from build123d import *

# Parameters (mm, degrees)
ESBO_O1_R                  = 25
EXTRUS_O1_DEPTH            = 8
EXTRUS_O2_DEPTH            = 8
CIRPATTERN1_COUNT          = 16
CORTE_EXTRUS_O2_DEPTH      = 10
CORTE_EXTRUS_O2_DEPTH_BACK = 37.138621999
ESBO_O5_R                  = 1.25
ESBO_O5_R_2                = 6
ESBO_O8_R                  = 23
ESBO_O8_R_2                = 19.75
CORTE_EXTRUS_O4_DEPTH      = 2
ESBO_O9_R                  = 9.5
CORTE_EXTRUS_O5_DEPTH      = 6
ESBO_O10_R                 = 1.5
CORTE_EXTRUS_O6_DEPTH      = 37.138621999


with BuildPart() as part:
    # Esboço1 → Extrusão1 (new body)
    with BuildSketch(Plane.XY):
        Circle(ESBO_O1_R)
    extrude(amount=-EXTRUS_O1_DEPTH)


with BuildPart() as body_2:
    # Esboço2 → Extrusão2 (new, through all)
    with BuildSketch(Plane(origin=(0, 0, -8), x_dir=(-1, 0, 0), z_dir=(0, 0, -1))):
        Polygon((0, 14.5), (2, 14.5), (2, 29.5), (-2, 29.5), (-2, 14.5), align=None)
    extrude(amount=-EXTRUS_O2_DEPTH)


with BuildPart() as cirpattern1_1:
    # CirPattern1: pattern copy
    add(body_2.part.rotate(Axis((0, 0, 0), (0, 0, 1)), 1 * 360 / CIRPATTERN1_COUNT))


with BuildPart() as cirpattern1_2:
    # CirPattern1: pattern copy
    add(body_2.part.rotate(Axis((0, 0, 0), (0, 0, 1)), 2 * 360 / CIRPATTERN1_COUNT))


with BuildPart() as cirpattern1_3:
    # CirPattern1: pattern copy
    add(body_2.part.rotate(Axis((0, 0, 0), (0, 0, 1)), 3 * 360 / CIRPATTERN1_COUNT))


with BuildPart() as cirpattern1_4:
    # CirPattern1: pattern copy
    add(body_2.part.rotate(Axis((0, 0, 0), (0, 0, 1)), 4 * 360 / CIRPATTERN1_COUNT))


with BuildPart() as cirpattern1_5:
    # CirPattern1: pattern copy
    add(body_2.part.rotate(Axis((0, 0, 0), (0, 0, 1)), 5 * 360 / CIRPATTERN1_COUNT))


with BuildPart() as cirpattern1_6:
    # CirPattern1: pattern copy
    add(body_2.part.rotate(Axis((0, 0, 0), (0, 0, 1)), 6 * 360 / CIRPATTERN1_COUNT))


with BuildPart() as cirpattern1_7:
    # CirPattern1: pattern copy
    add(body_2.part.rotate(Axis((0, 0, 0), (0, 0, 1)), 7 * 360 / CIRPATTERN1_COUNT))


with BuildPart() as cirpattern1_8:
    # CirPattern1: pattern copy
    add(body_2.part.rotate(Axis((0, 0, 0), (0, 0, 1)), 8 * 360 / CIRPATTERN1_COUNT))


with BuildPart() as cirpattern1_9:
    # CirPattern1: pattern copy
    add(body_2.part.rotate(Axis((0, 0, 0), (0, 0, 1)), 9 * 360 / CIRPATTERN1_COUNT))


with BuildPart() as cirpattern1_10:
    # CirPattern1: pattern copy
    add(body_2.part.rotate(Axis((0, 0, 0), (0, 0, 1)), 10 * 360 / CIRPATTERN1_COUNT))


with BuildPart() as cirpattern1_11:
    # CirPattern1: pattern copy
    add(body_2.part.rotate(Axis((0, 0, 0), (0, 0, 1)), 11 * 360 / CIRPATTERN1_COUNT))


with BuildPart() as cirpattern1_12:
    # CirPattern1: pattern copy
    add(body_2.part.rotate(Axis((0, 0, 0), (0, 0, 1)), 12 * 360 / CIRPATTERN1_COUNT))


with BuildPart() as cirpattern1_13:
    # CirPattern1: pattern copy
    add(body_2.part.rotate(Axis((0, 0, 0), (0, 0, 1)), 13 * 360 / CIRPATTERN1_COUNT))


with BuildPart() as cirpattern1_14:
    # CirPattern1: pattern copy
    add(body_2.part.rotate(Axis((0, 0, 0), (0, 0, 1)), 14 * 360 / CIRPATTERN1_COUNT))


with BuildPart() as cirpattern1_15:
    # CirPattern1: pattern copy
    add(body_2.part.rotate(Axis((0, 0, 0), (0, 0, 1)), 15 * 360 / CIRPATTERN1_COUNT))


with BuildPart() as part_1:
    add(part.part)

    # Combinar1: cut CirPattern1_15, body 2, CirPattern1_1, CirPattern1_2, CirPattern1_3, CirPattern1_4, CirPattern1_5, CirPattern1_6, CirPattern1_7, CirPattern1_8, CirPattern1_9, CirPattern1_10, CirPattern1_11, CirPattern1_12, CirPattern1_13, CirPattern1_14
    add(cirpattern1_15.part, mode=Mode.SUBTRACT)
    add(body_2.part, mode=Mode.SUBTRACT)
    add(cirpattern1_1.part, mode=Mode.SUBTRACT)
    add(cirpattern1_2.part, mode=Mode.SUBTRACT)
    add(cirpattern1_3.part, mode=Mode.SUBTRACT)
    add(cirpattern1_4.part, mode=Mode.SUBTRACT)
    add(cirpattern1_5.part, mode=Mode.SUBTRACT)
    add(cirpattern1_6.part, mode=Mode.SUBTRACT)
    add(cirpattern1_7.part, mode=Mode.SUBTRACT)
    add(cirpattern1_8.part, mode=Mode.SUBTRACT)
    add(cirpattern1_9.part, mode=Mode.SUBTRACT)
    add(cirpattern1_10.part, mode=Mode.SUBTRACT)
    add(cirpattern1_11.part, mode=Mode.SUBTRACT)
    add(cirpattern1_12.part, mode=Mode.SUBTRACT)
    add(cirpattern1_13.part, mode=Mode.SUBTRACT)
    add(cirpattern1_14.part, mode=Mode.SUBTRACT)

    # Esboço5 → Corte-extrusão2 (cut, two sides: drawn at the far end of the back side and taken through both)
    with BuildSketch(Plane(origin=(0, 0, -8), x_dir=(-1, 0, 0), z_dir=(0, 0, -1)).offset(-CORTE_EXTRUS_O2_DEPTH_BACK)):
        with Locations(Location((0, 11.5, 0), (0, 0, 180))):
            Circle(ESBO_O5_R)
        with Locations(Location((9.959292144, -5.75, 0), (0, 0, 180))):
            Circle(ESBO_O5_R)
        with Locations(Location((-9.959292144, -5.75, 0), (0, 0, 180))):
            Circle(ESBO_O5_R)
        with Locations(Location((0, 0, 0), (0, 0, 180))):
            Circle(ESBO_O5_R_2)
    extrude(amount=CORTE_EXTRUS_O2_DEPTH + CORTE_EXTRUS_O2_DEPTH_BACK, mode=Mode.SUBTRACT)

    # Esboço8 → Corte-extrusão4 (cut)
    with BuildSketch(Plane.XY):
        Circle(ESBO_O8_R)
        Circle(ESBO_O8_R_2, mode=Mode.SUBTRACT)
    extrude(amount=-CORTE_EXTRUS_O4_DEPTH, mode=Mode.SUBTRACT)

    # Esboço9 → Corte-extrusão5 (cut)
    with BuildSketch(Plane.XY):
        Circle(ESBO_O9_R)
    extrude(amount=-CORTE_EXTRUS_O5_DEPTH, mode=Mode.SUBTRACT)

    # Esboço10 → Corte-extrusão6 (cut, through all)
    with BuildSketch(Plane(origin=(0, 0, -8), x_dir=(-1, 0, 0), z_dir=(0, 0, -1))):
        with Locations((-4.29, -21.577671329)):
            Circle(ESBO_O10_R)
        with Locations((-21.577671329, 4.29)):
            Circle(ESBO_O10_R)
        with Locations((4.29, 21.577671329)):
            Circle(ESBO_O10_R)
        with Locations((21.577671329, -4.29)):
            Circle(ESBO_O10_R)
    extrude(amount=-CORTE_EXTRUS_O6_DEPTH, mode=Mode.SUBTRACT)


solid = part_1.part
Verification items for the finished model (mm, model axes). A direction names the side the tool comes from. Give positions to 0.01 mm unless a question says otherwise; leave off trailing zeros. Write each loop counter-clockwise with the first axis right and the second up, starting at its lowest first coordinate (ties: lowest second). Pieces come first, ordered by that corner, then holes. Notation, with made-up numbers: M -10.75,1 L 18.25,1 A15 ccw 18.25,26 Z; hole C 19,44 d3. An arc over 180 degrees is marked long. Put each result on its own line as item: value. Start each with the question number.
1. Scan lines: line 1 along Y through (x, z) = (0, -5.25); line 2 along Y through (x, z) = (0, -7); line 3 along X through (y, z) = (14, -3). Record each from-to range of solid material in increasing order. Write a range as [from, to].
2. Draft check along X on faces 4 (the face through (-18, 12, -2)), 5 (the face through (-23, 5, 0)). Enter one of: +X half, -X half, draft (parallel to the pull), parting line (faces both ways), or undercut.
3. Set-up check for faces 1 (the face through (-2, -20, -4)), 2 (the face through (-12.47, -15.3, -4.06)), 3 (the face through (12.807, 19.104, -0.986)): record each of +Z, -Z, +X, -X, +Y, -Y from which the full face is reachable in a straight line by a thin tool's end or side.
4. Go/stop test with flat-tipped pins: pin 1 Ø2.5 at (x, z) = (-17.5, -4) entering from -Y; pin 2 Ø1.2 at (x, z) = (-0.5, -4.5) entering from +Y; pin 3 Ø1.2 at (x, y) = (-4.5, -21) entering from +Z. Record where each tip stops, or that it passes through.
5. Section check A-A (y = 0). Record the cut outline in (x, z), and give its area (3 significant figures).
6. Section check B-B (x = 4.29). Give the number of separate pieces and of enclosed holes in the cut face, and give its area (3 significant figures).
7. Section check C-C (y = 13.5). Record the cut outline in (x, z).
Answer list:
1. line 1: [-14.5, -9.5], [9.5, 10.25], [12.75, 14.5]
1. line 2: [-14.5, -6], [6, 10.25], [12.75, 14.5]
1. line 3: [-20.71, -16.83], [-11.17, -7.96], [-4.09, 4.09], [7.96, 11.17], [16.83, 20.71]
2. face 4: undercut
2. face 5: draft
3. face 1: +Z, -Z, -Y
3. face 2: +Z, -Z
3. face 3: +Z
4. pin 1: y = -15.92
4. pin 2: y = 14.5
4. pin 3: z = -2
5. outline: M -14.5,-8 L -6,-8 L -6,-6 L -9.5,-6 L -9.5,0 L -14.5,0 Z; M 6,-8 L 14.5,-8 L 14.5,0 L 9.5,0 L 9.5,-6 L 6,-6 Z
5. area: 94.0 mm2
6. separate pieces: 5
6. enclosed holes: 0
6. area: 217 mm2
7. outline: M -21.04,-8 L -16.33,-8 L -16.33,-2 L -18.62,-2 L -18.62,0 L -21.04,0 Z; M -10.67,-8 L -7.76,-8 L -7.76,0 L -10.67,0 Z; M -5.3,-8 L 5.3,-8 L 5.3,0 L -5.3,0 Z; M 7.76,-8 L 10.67,-8 L 10.67,0 L 7.76,0 Z; M 16.33,-8 L 21.04,-8 L 21.04,0 L 18.62,0 L 18.62,-2 L 16.33,-2 Z
